Design review of the part built by this model. Coordinates are the model's own, in mm. Give positions to 0.01 mm unless a question says otherwise; leave off trailing zeros. Loops run counter-clockwise (first coordinate to the right, second up) from the corner with the lowest first, then second, coordinate; pieces in that order, holes last. Notation, with made-up numbers: M -0.75,81 L 25.25,81 A25 cw 25.25,95 Z; hole C 20.25,-2.5 d7. An arc over 180 degrees is marked long. Answer as CSV lines item,"result".
```python
from build123d import *

# Parameters (mm, degrees)
SKETCH1_W           = 45
SKETCH1_H           = 90
BOSS_EXTRUDE1_DEPTH = 2
SKETCH2_R           = 2
CUT_EXTRUDE1_DEPTH  = 10


with BuildPart() as part:
    # Sketch1 → Boss-Extrude1 (new body)
    with BuildSketch(Plane.XY):
        Polygon((200, 0), (-200, 0), (-200, -222.5), (-150.404334867, -275.82), (-130, -275.82), (-130, -222.5), (130, -222.5), (130, -275.82), (150.404334867, -275.82), (200, -222.5), align=None)
        with Locations((-165, -130)):
            Rectangle(SKETCH1_W, SKETCH1_H, mode=Mode.SUBTRACT)
        with Locations((165, -130)):
            Rectangle(SKETCH1_W, SKETCH1_H, mode=Mode.SUBTRACT)
    extrude(amount=BOSS_EXTRUDE1_DEPTH)

    # Sketch2 → Cut-Extrude1 (cut)
    with BuildSketch(Plane.XY.offset(2)):
        with Locations((-136.25, -238.82)):
            Circle(SKETCH2_R)
        with Locations((-136.25, -255.82)):
            Circle(SKETCH2_R)
        with Locations((136.25, -255.82)):
            Circle(SKETCH2_R)
        with Locations((136.25, -238.82)):
            Circle(SKETCH2_R)
    extrude(amount=-CUT_EXTRUDE1_DEPTH, mode=Mode.SUBTRACT)


solid = part.part
```
1. We need section A-A, the plane z = 0.65. Write out the cut boundary in (x, y), plus the area to 3 significant figures.
Answer block:
outline,"M -200,-222.5 L -150.4,-275.82 L -130,-275.82 L -130,-222.5 L 130,-222.5 L 130,-275.82 L 150.4,-275.82 L 200,-222.5 L 200,0 L -200,0 Z; hole M -187.5,-175 L -142.5,-175 L -142.5,-85 L -187.5,-85 Z; hole C -136.25,-255.82 d4; hole C -136.25,-238.82 d4; hole C 136.25,-255.82 d4; hole C 136.25,-238.82 d4; hole M 142.5,-175 L 187.5,-175 L 187.5,-85 L 142.5,-85 Z"
area,"85,700 mm²"
2. To check wall thickness, follow L1, parallel to Y at x = -136.25, z = 0.7; L2, parallel to X at y = -112, z = 0.1; L3, parallel to Y at x = -149.5, z = 0.9. State the ranges of each line that lie inside material, in increasing order. Write a range as [from, to].
Answer block:
L1,"[-275.82, -257.82], [-253.82, -240.82], [-236.82, 0]"
L2,"[-200, -187.5], [-142.5, 142.5], [187.5, 200]"
L3,"[-275.82, -175], [-85, 0]"
3. We need section C-C, the plane x = -175. Write out the cut boundary in (y, z), plus the area to 3 significant figures.
Answer block:
outline,"M -249.38,0 L -175,0 L -175,2 L -249.38,2 Z; M -85,0 L 0,0 L 0,2 L -85,2 Z"
area,"319 mm²"
4. We need section D-D, the plane x = -101. Write out the cut boundary in (y, z), plus the area to 3 significant figures.
Answer block:
outline,"M -222.5,0 L 0,0 L 0,2 L -222.5,2 Z"
area,"445 mm²"
5. We need section B-B, the plane y = -249. Write out the cut boundary in (x, z), plus the area to 3 significant figures.
Answer block:
outline,"M -175.35,0 L -130,0 L -130,2 L -175.35,2 Z; M 130,0 L 175.35,0 L 175.35,2 L 130,2 Z"
area,"181 mm²"
6. For P1, Ø0.6, axis at y = -241.5, z = 0.5, coming from the -X side; P2, Ø0.6, axis at x = -162.5, z = 1.5, coming from the -Y side; P3, Ø1, axis at y = -262.5, z = 1.5, coming from the +X side, all flat-tipped, find the tip position at first contact; note any pin that passes through.
Answer block:
P1,"x = -182.61"
P2,"y = -263.14"
P3,"x = 163.26"
